Geometry: see drawing. Coordinates: mm, zero at the bounding-box minimum. A direction names the side the tool comes from. Coordinates: 2 decimals unless noted, no trailing zeros. Write each loop counter-clockwise with the first axis right and the second up, starting at its lowest first coordinate (ties: lowest second). Pieces come first, ordered by that corner, then holes. Notation, with made-up numbers: M 59.5,-24.5 L 95.5,-24.5 A24 ccw 95.5,4.5 Z; hole C -6,55.5 d4. An arc over 180 degrees is marked long. Write item = value, one per line. Start each with the question number.
1. Pin query (flat end, axial travel): pin 1 Ø8 at (y, z) = (30.5, 11) entering from -X; pin 2 Ø1 at (y, z) = (75.5, 65.5) entering from -X; pin 3 Ø14 at (x, z) = (4.5, 36) entering from +Y; pin 4 Ø23 at (y, z) = (66, 27) entering from +X. Return the tip coordinate at first contact, or that it passes through.
2. Section query D-D (z = 38.1). Output: boundary loops of the cut face in (x, y).
3. Section query B-B (x = 63.5). Output: boundary loops of the cut face in (y, z).
4. Section query A-A (y = 50.8). Output: boundary loops of the cut face in (x, z).
5. Access query for the marked faces 5, 6, 7, 8 and 9. Directions: +Z, -Z, +X, -X, +Y, -Y. A direction counts if a zero-diameter tool reaches every point of the face in a straight line with its end or side. Return the directions, or none.
6. Line query: line 1 along Y through (x, z) = (63.5, 53.5); line 2 along X through (y, z) = (50, 39) (1 decimal); line 3 along Y through (x, z) = (63, 33). Output: solid intervals per line, ascending.
7. Pull-direction query (X, two-part tool) for the marked faces 1, 2, 3 and 4; classes: pulls with the +X half, pulls with the -X half, needs draft (parallel to the pull), parting line crosses it, or undercut.
8. Section query C-C (z = 61). Output: boundary loops of the cut face in (x, y), then the cut area to 3 significant figures.
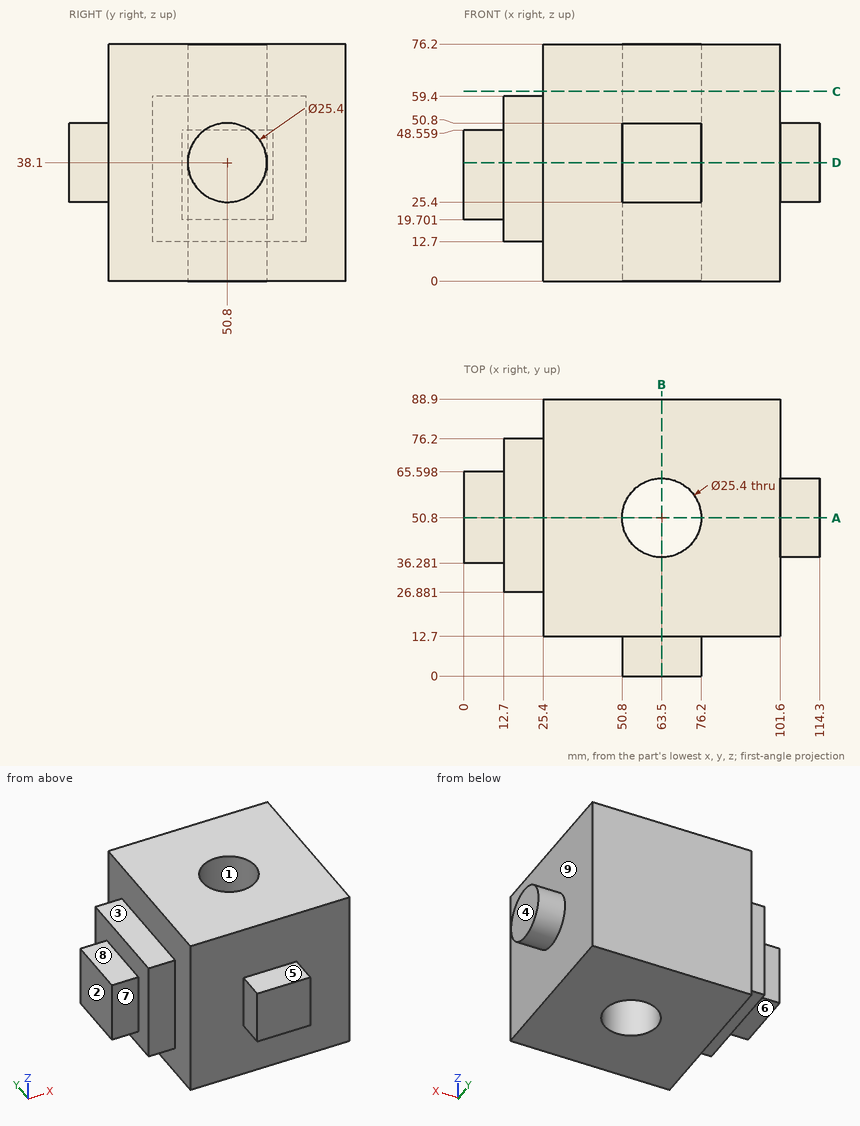
Results are:
q1.pin_1 = 12.7
q1.pin_2 = 25.4
q1.pin_3 = 65.6
q1.pin_4 = 114.3
q2.outline = M 0,36.28 L 12.7,36.28 L 12.7,26.88 L 25.4,26.88 L 25.4,12.7 L 50.8,12.7 L 50.8,0 L 76.2,0 L 76.2,12.7 L 101.6,12.7 L 101.6,38.1 L 114.3,38.1 L 114.3,63.5 L 101.6,63.5 L 101.6,88.9 L 25.4,88.9 L 25.4,76.2 L 12.7,76.2 L 12.7,65.6 L 0,65.6 Z; hole C 63.5,50.8 d25.4
q3.outline = M 0,25.4 L 12.7,25.4 L 12.7,0 L 38.1,0 L 38.1,76.2 L 12.7,76.2 L 12.7,50.8 L 0,50.8 Z; M 63.5,0 L 88.9,0 L 88.9,76.2 L 63.5,76.2 Z
q4.outline = M 0,19.7 L 12.7,19.7 L 12.7,12.7 L 25.4,12.7 L 25.4,0 L 50.8,0 L 50.8,76.2 L 25.4,76.2 L 25.4,59.4 L 12.7,59.4 L 12.7,48.56 L 0,48.56 Z; M 76.2,0 L 101.6,0 L 101.6,25.4 L 114.3,25.4 L 114.3,50.8 L 101.6,50.8 L 101.6,76.2 L 76.2,76.2 Z
q5.face_5 = +Z, +X, -X, -Y
q5.face_6 = -Z, -X, +Y, -Y
q5.face_7 = +Z, -Z, -X, -Y
q5.face_8 = +Z, -X, +Y, -Y
q5.face_9 = +X
q6.line_1 = 12.7 to 38.1, 63.5 to 88.9
q6.line_2 = 0 to 50.8, 76.2 to 114.3
q6.line_3 = 0 to 38.11, 63.49 to 88.9
q7.face_1 = undercut
q7.face_2 = pulls with the -X half
q7.face_3 = needs draft
q7.face_4 = pulls with the +X half
q8.outline = M 25.4,12.7 L 101.6,12.7 L 101.6,88.9 L 25.4,88.9 Z; hole C 63.5,50.8 d25.4
q8.area = 5,300 mm^2
